CAD build for the part. Positions are in the model's coordinates, mm. A direction names the side the tool comes from. Coordinates: 2 decimals unless noted, no trailing zeros. Loops run counter-clockwise (first coordinate to the right, second up) from the corner with the lowest first, then second, coordinate; pieces in that order, holes last. Notation, with made-up numbers: M 32,-26.5 L 79,-26.5 A30 cw 79,5.5 Z; hole C 65.25,64 d5. An arc over 180 degrees is marked long. Answer as a JSON object with one key per item and string values. Group by question number.
```python
from build123d import *

# Parameters (mm, degrees)
BOSS_EXTRUDE1_DEPTH = 40
SKETCH2_R           = 9
CUT_EXTRUDE8_DEPTH  = 2
SKETCH6_R           = 3.25
CUT_EXTRUDE9_DEPTH  = 61.695963622
SKETCH7_R           = 1.7
CUT_EXTRUDE10_DEPTH = 61
SKETCH8_R           = 1.7
CUT_EXTRUDE11_DEPTH = 61.547502013
BOSS_EXTRUDE3_DEPTH = 3


with BuildPart() as part:
    # Sketch1 → Boss-Extrude1 (new body)
    with BuildSketch(Plane(origin=(0, 0, 0), x_dir=(0, 0, -1), z_dir=(1, 0, 0))):
        Polygon((0, 0), (40, 0), (40, 15), (40, 35), (29, 35), (29, 15), (0, 15), align=None)
    extrude(amount=BOSS_EXTRUDE1_DEPTH)

    # Sketch2 → Cut-Extrude8 (cut)
    with BuildSketch(Plane(origin=(0, 15, 0), x_dir=(1, 0, 0), z_dir=(0, 1, 0))):
        with Locations(Location((20, 14.5, 0), (0, 0, 270))):
            Circle(SKETCH2_R)
    extrude(amount=-CUT_EXTRUDE8_DEPTH, mode=Mode.SUBTRACT)

    # Sketch6 → Cut-Extrude9 (cut, through all)
    with BuildSketch(Plane(origin=(0, 13, 0), x_dir=(1, 0, 0), z_dir=(0, 1, 0))):
        with Locations(Location((20, 14.5, 0), (0, 0, 270))):
            Circle(SKETCH6_R)
    extrude(amount=-CUT_EXTRUDE9_DEPTH, mode=Mode.SUBTRACT)

    # Sketch7 → Cut-Extrude10 (cut, through all)
    with BuildSketch(Plane(origin=(0, 15, 0), x_dir=(1, 0, 0), z_dir=(0, 1, 0))):
        with Locations(Location((31, 14.5, 0), (0, 0, 270))):
            Circle(SKETCH7_R)
        with Locations(Location((20, 25.5, 0), (0, 0, 270))):
            Circle(SKETCH7_R)
        with Locations(Location((9, 14.5, 0), (0, 0, 270))):
            Circle(SKETCH7_R)
        with Locations(Location((20, 3.5, 0), (0, 0, 270))):
            Circle(SKETCH7_R)
    extrude(amount=-CUT_EXTRUDE10_DEPTH, mode=Mode.SUBTRACT)

    # Sketch8 → Cut-Extrude11 (cut, through all)
    with BuildSketch(Plane.XY.offset(-29)):
        with Locations((35, 30)):
            Circle(SKETCH8_R)
        with Locations((35, 20)):
            Circle(SKETCH8_R)
        with Locations((5, 30)):
            Circle(SKETCH8_R)
        with Locations((5, 20)):
            Circle(SKETCH8_R)
    extrude(amount=-CUT_EXTRUDE11_DEPTH, mode=Mode.SUBTRACT)

    # Sketch9 → Boss-Extrude3 (add)
    with BuildSketch(Plane(origin=(40, 0, 0), x_dir=(0, 0, -1), z_dir=(1, 0, 0))):
        Polygon((29, 25), (29, 15), (19, 15), align=None)
    boss_extrude3 = extrude(amount=-BOSS_EXTRUDE3_DEPTH)

    # Mirror3: Boss-Extrude3 across plane
    add(boss_extrude3.mirror(Plane.ZY.offset(-20)))


solid = part.part
```
Item 1: Pin check, flat tips, straight feed: pin 1 (3 mm diameter, centred on x = 11, z = -6.5, fed in from +Y); pin 2 (6 mm diameter, centred on x = 24.5, y = 30, fed in from +Z). Stop position of each tip, or through.
Item 2: Tool access for faces 1 (the cylindrical face through (29.5, 7.6, -13.7)), 2 (the flat face through (11, 15, -11)), 3 (the cylindrical face through (22.703, 14.014, -5.916)): list every direction of +Z, -Z, +X, -X, +Y, -Y with a clear straight run to the whole face (end or side of a thin tool).
Item 3: Pull direction Y, two halves, no side cores. Call faces 4 (the flat face through (3, 18, -26)), 5 (the flat face through (20, 13, -11)), 6 (the flat face through (20, 0, -20)), 7 (the cylindrical face through (34.63, 28.34, -34.42)): released by +Y, released by -Y, zero draft, split by the parting line, or undercut.
Item 4: Slice it at A-A, the plane x = 9. Write the cut outline in (y, z), then the cut area to 3 significant figures.
Item 5: Drill centre lines: L1, parallel to X at y = 6.25, z = -14.5; L2, parallel to Y at x = 5, z = -32.5; L3, parallel to Y at x = 35.5, z = -38. Where is each one in solid material? Low to high. Write a range as from..to.
Item 6: Slice it at B-B, the plane y = 20. Write the cut outline in (x, z).
Item 7: Slice it at C-C, the plane z = -3.5. Write the cut outline in (x, y), then the cut area to 3 significant figures.
Item 8: Slice it at D-D, the plane x = 20. Write the cut outline in (y, z).
Computed:
{
 "1": {"pin 1": "y = 15", "pin 2": "z = -29"},
 "2": {"face 1": "+Y, -Y", "face 2": "+Z, +Y", "face 3": "+Y"},
 "3": {"face 4": "zero draft", "face 5": "released by +Y", "face 6": "released by -Y", "face 7": "undercut"},
 "4": {"outline": "M 0,-40 L 35,-40 L 35,-29 L 15,-29 L 15,-16.2 L 0,-16.2 Z; M 0,-12.8 L 15,-12.8 L 15,0 L 0,0 Z", "area": "769 mm2"},
 "5": {"L1": "0..7.3, 10.7..16.75, 23.25..29.3, 32.7..40", "L2": "0..18.3, 21.7..28.3, 31.7..35", "L3": "0..18.38, 21.62..28.38, 31.62..35"},
 "6": {"outline": "M 0,-40 L 3.3,-40 L 3.3,-29 L 3,-29 L 3,-24 L 0,-24 Z; M 6.7,-40 L 33.3,-40 L 33.3,-29 L 6.7,-29 Z; M 36.7,-40 L 40,-40 L 40,-24 L 37,-24 L 37,-29 L 36.7,-29 Z"},
 "7": {"outline": "M 0,0 L 18.3,0 L 18.3,15 L 0,15 Z; M 21.7,0 L 40,0 L 40,15 L 21.7,15 Z", "area": "549 mm2"},
 "8": {"outline": "M 0,-40 L 35,-40 L 35,-29 L 15,-29 L 15,-27.2 L 0,-27.2 Z; M 0,-23.8 L 15,-23.8 L 15,-23.5 L 13,-23.5 L 13,-17.75 L 0,-17.75 Z; M 0,-11.25 L 13,-11.25 L 13,-5.5 L 15,-5.5 L 15,-5.2 L 0,-5.2 Z; M 0,-1.8 L 15,-1.8 L 15,0 L 0,0 Z"}
}
